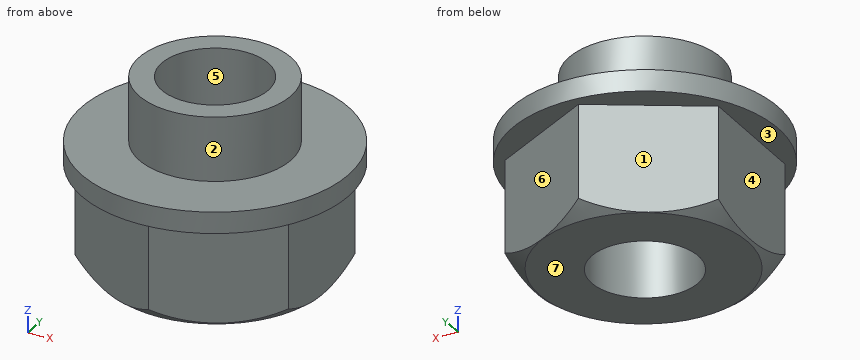
Autodesk Inventor part; units mm, degrees
ref_plane "YZ Plane" through (0, 0, 0) normal (1, 0, 0) x (0, 1, 0)
ref_plane "XZ Plane" through (0, 0, 0) normal (0, 1, 0) x (-1, 0, 0)
ref_plane "XY Plane" through (0, 0, 0) normal (0, 0, 1) x (1, 0, 0)
sketch "Sketch1" plane through (0, 0, 0) normal (0, 0, 1) x (1, 0, 0)
  line L0 (5, -2.8868) -> (0, -5.7735)
  line L1 (0, -5.7735) -> (-5, -2.8868)
  line L2 (-5, -2.8868) -> (-5, 2.8868)
  line L3 (-5, 2.8868) -> (0, 5.7735)
  line L4 (0, 5.7735) -> (5, 2.8868)
  line L5 (5, 2.8868) -> (5, -2.8868)
  point P0 (0, 0)
  point P1 (0, 0)
  dimension "d0" = 10
extrude "Extrusion1" add sketch "Sketch1" along normal blind 5
sketch "Sketch2" plane through (0, 0, 5) normal (0, 0, 1) x (1, 0, 0)
  circle A0 centre (0, 0) radius 6.25
  dimension "d3" = 12.5
extrude "Extrusion2" add sketch "Sketch2" along normal blind 1
sketch "Sketch3" plane through (0, 0, 6) normal (0, 0, 1) x (1, 0, 0)
  circle A0 centre (0, 0) radius 6.25
  circle A1 centre (0, 0) radius 3.56
  dimension "d6" = 7.12
extrude "Extrusion3" add sketch "Sketch3" along normal blind 3 contours A1
sketch "Sketch4" plane through (0, 0, 9) normal (0, 0, 1) x (1, 0, 0)
  circle A0 centre (0, 0) radius 3.56
  circle A1 centre (0, 0) radius 2.5
  dimension "d9" = 5
extrude "Extrusion4" cut sketch "Sketch4" against normal up to next contours A1
sketch "Sketch5" plane through (0, 0, 0) normal (1, 0, 0) x (0, 1, 0)
  arc A0 (0.1187, -1.552) -> (0.1187, 15.367) centre (0.1187, 6.9075) ccw
  arc A1 (0.1187, -2.8398) -> (0.1187, 16.6548) centre (0.1187, 6.9075) ccw
  line L0 (0.1187, -2.8398) -> (0.1187, 16.6548)
  point P0 (0, 0)
revolve "Revolution1" cut sketch "Sketch5" angle 360 about axis through (0, 0.1187, -2.8398) along (0, 0, 1) contours A0 L0 A1
properties part number "Eccentric Spacer 6mm"
CAD build for the part. Positions are in the model's coordinates, mm. Face numbers are marked on the shaded views. A direction names the side the tool comes from. Round coordinates to 2 decimals unless told otherwise and drop trailing zeros. Order: outer loops, then holes, each group sorted by start corner. A loop starts at its lowest first (then second) coordinate and runs counter-clockwise, first axis right, second up. Notation, with made-up numbers: (15.5, 58.25) -> (23.5, 58.25) arc R26 ccw to (23.5, 75.25) -> close; hole circle Ø11 at (87, -29.75). An arc over 180 degrees is marked (long way). Write item = value, one per line.
(1) Cut at B-B (z = 3.75). Write the cut outline in (x, y).
Answers follow:
outline = (-5, -2.89) -> (0, -5.77) -> (5, -2.89) -> (5, 2.89) -> (0, 5.77) -> (-5, 2.89) -> close; hole circle Ø5 at (0, 0)
(2) Cut at A-A (x = 0.25). Write the cut outline in (y, z) (1 decimal).
Answers follow:
outline = (-6.2, 5) -> (-5.6, 5) -> (-5.6, 0.7) arc R8.5 ccw to (-4.8, 0) -> (-2.5, 0) -> (-2.5, 9) -> (-3.6, 9) -> (-3.6, 6) -> (-6.2, 6) -> close; (2.5, 0) -> (5, 0) arc R8.5 ccw to (5.6, 0.5) -> (5.6, 5) -> (6.2, 5) -> (6.2, 6) -> (3.6, 6) -> (3.6, 9) -> (2.5, 9) -> close
(3) 3-axis set-ups, long thin cutter, end or side, ignore diameter. For the marked faces 1, 2, 3 and 4: which of +Z, -Z, +X, -X, +Y, -Y reach the whole face in a straight line?
Answers follow:
face_1 = -Z, -X, +Y
face_2 = +Z
face_3 = -Z
face_4 = -Z, -X, +Y, -Y
(4) Drill centre lines: L1, parallel to Y at x = 0, z = 5.25; L2, parallel to Z at x = -4, y = -1.5; L3, parallel to Y at x = -1.5, z = 2.75. Where is each one in solid material? Low to high.
Answers follow:
L1 = -6.25 to -2.5, 2.5 to 6.25
L2 = 0 to 6
L3 = -4.91 to -2, 2 to 4.91
(5) Cut at D-D (y = -4.25). Write the cut outline in (x, z), plus the area to 3 significant figures.
Answers follow:
outline = (-4.58, 5) -> (-2.64, 5) -> (-2.64, 0.16) arc R7.24 ccw to (-2.18, 0) -> (2.18, 0) arc R7.24 ccw to (2.64, 0.16) -> (2.64, 5) -> (4.58, 5) -> (4.58, 6) -> (-4.58, 6) -> close
area = 35.5 mm²
(6) Pull direction Y, two halves, no side cores. Call the marked faces 5, 6 and 7: +Y half, -Y half, draft (parallel to the pull), parting line (faces both ways), or undercut.
Answers follow:
face_5 = undercut
face_6 = +Y half
face_7 = draft
(7) Flat gauge pins, fed straight in: P1, Ø2, axis at x = -3.5, z = 5.5, coming from the +Y side; P2, Ø1.5, axis at y = -4.5, z = 4, coming from the -X side; P3, Ø2.5, axis at y = -1, z = 1.5, coming from the -X side. Where does each tip first touch, or does it go through?
Answers follow:
P1 = 5.73
P2 = -3.5
P3 = -5
(8) Cut at C-C (y = -2). Write the cut outline in (x, z).
Answers follow:
outline = (-5.92, 5) -> (-5, 5) -> (-5, 0.42) arc R8.19 ccw to (-4.4, 0) -> (-1.5, 0) -> (-1.5, 9) -> (-2.95, 9) -> (-2.95, 6) -> (-5.92, 6) -> close; (1.5, 0) -> (4.4, 0) arc R8.19 ccw to (5, 0.42) -> (5, 5) -> (5.92, 5) -> (5.92, 6) -> (2.95, 6) -> (2.95, 9) -> (1.5, 9) -> close
